from build123d import *

# Parameters (mm, degrees)
SKETCH1_R                                       = 56.4
SKETCH1_R_2                                     = 44.4
BOSS_EXTRUDE1_DEPTH                             = 8.5
CSK_FOR_M5_FLAT_HEAD_MACHINE_SCREW1_D           = 5.5
CSK_FOR_M5_FLAT_HEAD_MACHINE_SCREW1_DEPTH       = 30
CSK_FOR_M5_FLAT_HEAD_MACHINE_SCREW1_CSINK_D     = 10.4
CSK_FOR_M5_FLAT_HEAD_MACHINE_SCREW1_CSINK_ANGLE = 90
CSK_FOR_M5_FLAT_HEAD_MACHINE_SCREW1_TIP         = 1.652366702


with BuildPart() as part:
    # Sketch1 → Boss-Extrude1 (new body)
    with BuildSketch(Plane(origin=(0, 0, 0), x_dir=(1, 0, 0), z_dir=(0, 1, 0))):
        with Locations(Location((0, 0, 0), (0, 0, 270))):
            Circle(SKETCH1_R)
        with Locations(Location((0, 0, 0), (0, 0, 270))):
            Circle(SKETCH1_R_2, mode=Mode.SUBTRACT)
    extrude(amount=BOSS_EXTRUDE1_DEPTH)

    # CSK for M5 Flat Head Machine Screw1
    with Locations(Plane(origin=(0, 8.5, 0), x_dir=(1, 0, 0), z_dir=(0, 1, 0))):
        with Locations((35.638181772, 35.638181772), (35.638181772, -35.638181772), (-35.638181772, -35.638181772), (-35.638181772, 35.638181772)):
            CounterSinkHole(CSK_FOR_M5_FLAT_HEAD_MACHINE_SCREW1_D / 2, CSK_FOR_M5_FLAT_HEAD_MACHINE_SCREW1_CSINK_D / 2, depth=CSK_FOR_M5_FLAT_HEAD_MACHINE_SCREW1_DEPTH, counter_sink_angle=CSK_FOR_M5_FLAT_HEAD_MACHINE_SCREW1_CSINK_ANGLE)
            with Locations((0, 0, -(CSK_FOR_M5_FLAT_HEAD_MACHINE_SCREW1_DEPTH + CSK_FOR_M5_FLAT_HEAD_MACHINE_SCREW1_TIP / 2))):  # 118° drill point
                Cone(0, CSK_FOR_M5_FLAT_HEAD_MACHINE_SCREW1_D / 2, CSK_FOR_M5_FLAT_HEAD_MACHINE_SCREW1_TIP, mode=Mode.SUBTRACT)


solid = part.part
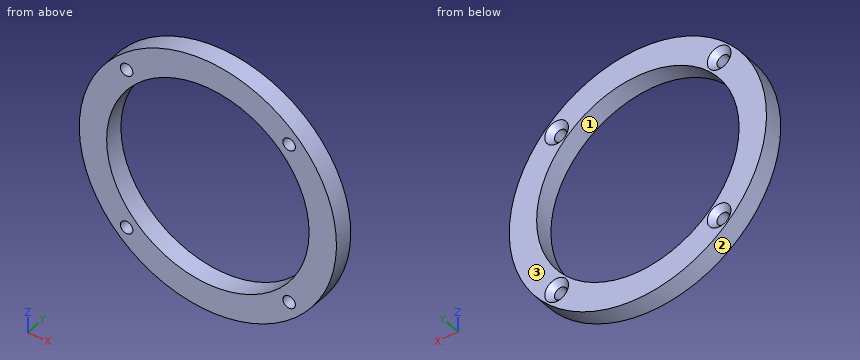
Here's how the part is built. I have some questions about the finished solid (model axes, mm). Face numbers are marked on the shaded views. Coordinates: 2 decimals unless noted, no trailing zeros. Loops run counter-clockwise (first coordinate to the right, second up) from the corner with the lowest first, then second, coordinate; pieces in that order, holes last. Notation, with made-up numbers: (85, 44) -> (91, 44) arc R14 ccw to (91, 52) -> close; hole circle Ø1 at (52, 13). An arc over 180 degrees is marked (long way). Use one line per item in the form item = value. Start each with the question number.
(1) If we section it at A-A (x = 0): Please give me the cut outline in (y, z), then the cut area to 3 significant figures.
(2) If we section it at C-C (y = 1.75): Please give me the cut outline in (x, z).
(3) If we section it at B-B (z = 0): Please give me the cut outline in (x, y).
(4) Please list where these lines run through material, in increasing order: line 1 along Z through (x, y) = (-39, 8.25); line 2 along X through (y, z) = (2, 0); line 3 along Z through (x, y) = (-36.5, 5).
(5) We'd pull the mould along X, two halves only. Please class the marked faces 1, 2 and 3: pulls with the +X half, pulls with the -X half, needs draft (parallel to the pull), parting line crosses it, or undercut.
(6) Will these pins go through, and if not, where does the flat tip stop? pin 1 (4 mm diameter, centred on y = 2, z = -21.5, fed in from +X); pin 2 (9 mm diameter, centred on x = -35.64, z = -35.64, fed in from +Y).
Verdict:
q1.outline = (0, -56.4) -> (8.5, -56.4) -> (8.5, -44.4) -> (0, -44.4) -> close; (0, 44.4) -> (8.5, 44.4) -> (8.5, 56.4) -> (0, 56.4) -> close
q1.area = 204 mm²
q2.outline = circle Ø112.8 at (0, 0); hole circle Ø88.8 at (0, 0); hole circle Ø5.5 at (-35.64, -35.64); hole circle Ø5.5 at (-35.64, 35.64); hole circle Ø5.5 at (35.64, -35.64); hole circle Ø5.5 at (35.64, 35.64)
q3.outline = (-56.4, 0) -> (-44.4, 0) -> (-44.4, 8.5) -> (-56.4, 8.5) -> close; (44.4, 0) -> (56.4, 0) -> (56.4, 8.5) -> (44.4, 8.5) -> close
q4.line_1 = -40.74 to -39.27, -32 to -21.22, 21.22 to 32, 39.27 to 40.74
q4.line_2 = -56.4 to -44.4, 44.4 to 56.4
q4.line_3 = -43 to -38.25, -33.03 to -25.28, 25.28 to 33.03, 38.25 to 43
q5.face_1 = undercut
q5.face_2 = parting line crosses it
q5.face_3 = needs draft
q6.pin_1 = 52.92
q6.pin_2 = 7.8
